```python
from build123d import *

# Parameters (mm, degrees)
CYLINDER396_R     = 1.7
CYLINDER396_DEPTH = 10
PRISM028_DEPTH    = 2.4
CYLINDER402_R     = 8
CYLINDER402_DEPTH = 3
CYLINDER400_R     = 4
CYLINDER400_DEPTH = 3


with BuildPart() as cone006:
    # Cone005 → Cone005 (revolve)
    with BuildSketch(Plane(origin=(0, 0, 85), x_dir=(1, 0, 0), z_dir=(0, -1, 0))):
        Polygon((0, 0), (21, 0), (5, 41), (0, 41), align=None)
    revolve(axis=Axis((0, 0, 85), (0, 0, 1)))


with BuildPart() as cylinder396:
    # Cylinder396 → Cylinder396 (new body)
    with BuildSketch(Plane.XY.offset(120)):
        Circle(CYLINDER396_R)
    extrude(amount=CYLINDER396_DEPTH)


with BuildPart() as fusion075:
    # Prism028 → Prism028 (new body)
    with BuildSketch(Plane.XY.offset(123.6)):
        Polygon((3.3, 0), (1.65, 2.857884), (-1.65, 2.857884), (-3.3, 0), (-1.65, -2.857884), (1.65, -2.857884), align=None)
    extrude(amount=PRISM028_DEPTH)

    # Fusion076: union Cylinder396
    add(cylinder396.part)


with BuildPart() as cylinder402:
    # Cylinder402 → Cylinder402 (new body)
    with BuildSketch(Plane.XY.offset(120)):
        Circle(CYLINDER402_R)
    extrude(amount=CYLINDER402_DEPTH)


with BuildPart() as support_antenna:
    # Cylinder400 → Cylinder400 (new body)
    with BuildSketch(Plane.XY.offset(123)):
        Circle(CYLINDER400_R)
    extrude(amount=CYLINDER400_DEPTH)

    # Fusion078: union Cylinder402
    add(cylinder402.part)

    # Cut210: cut Fusion075
    add(fusion075.part, mode=Mode.SUBTRACT)

    # Common005: intersect Cone006
    add(cone006.part, mode=Mode.INTERSECT)


solid = support_antenna.part
```
Design review of the part built by this model. Coordinates are the model's own, in mm. A direction names the side the tool comes from. Give positions to 0.01 mm unless a question says otherwise; leave off trailing zeros. Loops run counter-clockwise (first coordinate to the right, second up) from the corner with the lowest first, then second, coordinate; pieces in that order, holes last. Notation, with made-up numbers: (54, -16.75) -> (86, -16.75) arc R9 cw to (86, -8.75) -> close; hole circle Ø2 at (81, 70.25). An arc over 180 degrees is marked (long way). One line per item, written item: value.
Q1. For pin 1 Ø3 at (x, z) = (4.5, 122) entering from +Y; pin 2 Ø1.5 at (y, z) = (6, 122) entering from -X; pin 3 Ø1 at (x, z) = (-4, 124.5) entering from +Y, all flat-tipped, find the tip position at first contact; note any pin that passes through.
Numbers:
pin 1: stops at y = 6.07
pin 2: stops at x = -4.05
pin 3: stops at y = 1.94
Q2. We need section D-D on z = 121.35. Give the boundary of the cut face in (x, y), and give its area (3 significant figures).
Numbers:
outline: circle Ø13.63 at (0, 0); hole circle Ø3.4 at (0, 0)
area: 137 mm^2
Q3. Machinability: for faces 1 (the cylindrical face through (-0.37, -1.66, 121.77)), 2 (the flat face through (1.4, 1.3, 123.6)), which of the approach directions +Z, -Z, +X, -X, +Y, -Y give a long, thin tool a straight path to every point of the face, cutting with its end or side? Answer none if there is none.
Numbers:
face 1: +Z, -Z
face 2: +Z
Q4. We need section C-C on z = 122.5. Give the boundary of the cut face in (x, y), and give its area (3 significant figures).
Numbers:
outline: circle Ø12.73 at (0, 0); hole circle Ø3.4 at (0, 0)
area: 118 mm^2
Q5. Draft analysis for pull direction X (two halves, no side actions). For faces 3 (the flat face through (-2.463, 1.449, 124.783)), 4 (the cylindrical face through (-0.867, -3.905, 124.479)), 5 (the flat face through (4, -1.3, 123)), state which applies: pulls with the +X half, pulls with the -X half, needs draft (parallel to the pull), parting line crosses it, or undercut.
Numbers:
face 3: undercut
face 4: parting line crosses it
face 5: needs draft
Q6. For L1, parallel to Z at x = -0.75, y = 4.75; L2, parallel to X at y = 0.25, z = 122.4; L3, parallel to X at y = -0.5, z = 120.35, list the stretches that pass through material, from the lowest coordinate up.
Numbers:
L1: z = 120 to 123
L2: x = -6.4 to -1.68, 1.68 to 6.4
L3: x = -7.19 to -1.62, 1.62 to 7.19
Q7. We need section B-B on z = 125.65. Give the boundary of the cut face in (x, y), and give its area (3 significant figures).
Numbers:
outline: circle Ø8 at (0, 0); hole (-3.3, 0) -> (-1.65, -2.86) -> (1.65, -2.86) -> (3.3, 0) -> (1.65, 2.86) -> (-1.65, 2.86) -> close
area: 22.0 mm^2
Q8. We need section A-A on x = 0. Give the boundary of the cut face in (y, z), and give its area (3 significant figures).
Numbers:
outline: (-7.34, 120) -> (-1.7, 120) -> (-1.7, 123.6) -> (-2.86, 123.6) -> (-2.86, 126) -> (-4, 126) -> (-4, 123) -> (-6.17, 123) -> close; (1.7, 120) -> (7.34, 120) -> (6.17, 123) -> (4, 123) -> (4, 126) -> (2.86, 126) -> (2.86, 123.6) -> (1.7, 123.6) -> close
area: 38.6 mm^2
